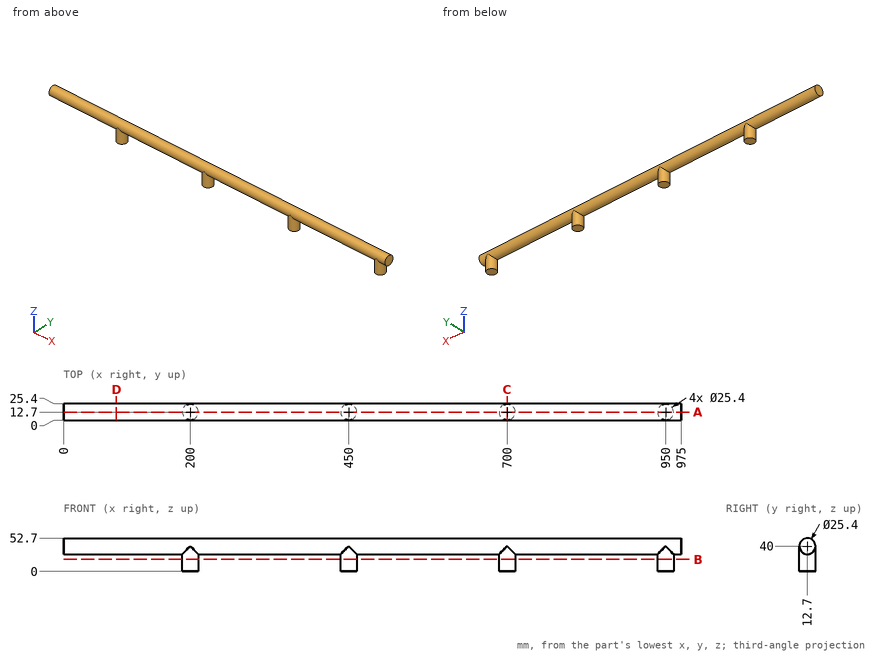
Design review of the part shown in the three views and the two pictorial views. Dimensions are in mm from the part's minimum x, y and z. Give positions to 0.01 mm unless a question says otherwise; leave off trailing zeros. Order: outer loops, then holes, each group sorted by start corner. A loop starts at its lowest first (then second) coordinate and runs counter-clockwise, first axis right, second up. Notation, with made-up numbers: M 13.5,71 L 41.5,71 A34 ccw 41.5,110 Z; hole C 37.5,56.25 d10. An arc over 180 degrees is marked long. Answer in a Markdown table with one row per item. Add a question column.
(1) Consider section C-C on x = 700. State the section outline as (y, z) points, and give its area (3 significant figures).
(2) Consider section A-A on y = 12.7. State the section outline as (x, z) points, and give its area (3 significant figures).
(3) For pin 1 (6 mm diameter, centred on x = 280, z = 43.5, fed in from +Y); pin 2 (4 mm diameter, centred on x = 542, y = 7, fed in from -Z); pin 3 (4 mm diameter, centred on x = 265.5, z = 45.5, fed in from -Y), all flat-tipped, find the tip position at first contact; note any pin that passes through.
(4) Wall thickness on probe 1 along X at (y, z) = (12, 20); probe 2 along X at (y, z) = (3, 29.5); probe 3 along Z at (x, y) = (685, 11): over which ranges is each line inside the solid? List them lowest first. Write a range as [from, to].
(5) Consider section B-B on z = 19. State the section outline as (x, y) points, and give its area (3 significant figures).
(6) Consider section D-D on x = 83.5. State the section outline as (y, z) points, and give its area (3 significant figures).
Evaluation:
| question | item | result |
|---|---|---|
| 1 | outline | M 0,0 L 25.4,0 L 25.4,40 A12.7 ccw 0,40 Z |
| 1 | area | 1,270 mm^2 |
| 2 | outline | M 0,27.3 L 187.3,27.3 L 187.3,0 L 212.7,0 L 212.7,27.3 L 437.3,27.3 L 437.3,0 L 462.7,0 L 462.7,27.3 L 687.3,27.3 L 687.3,0 L 712.7,0 L 712.7,27.3 L 937.3,27.3 L 937.3,0 L 962.7,0 L 962.7,27.3 L 975,27.3 L 975,52.7 L 0,52.7 Z |
| 2 | area | 27,500 mm^2 |
| 3 | pin 1 | stops at y = 25.39 |
| 3 | pin 2 | stops at z = 27.85 |
| 3 | pin 3 | stops at y = 0.49 |
| 4 | probe 1 | x = [187.32, 212.68], [437.32, 462.68], [687.32, 712.68], [937.32, 962.68] |
| 4 | probe 2 | x = [191.8, 208.2], [441.8, 458.2], [691.8, 708.2], [941.8, 958.2] |
| 4 | probe 3 | z = [27.41, 52.59] |
| 5 | outline | C 200,12.7 d25.4; C 450,12.7 d25.4; C 700,12.7 d25.4; C 950,12.7 d25.4 |
| 5 | area | 2,030 mm^2 |
| 6 | outline | C 12.7,40 d25.4 |
| 6 | area | 507 mm^2 |
